```python
from build123d import *

# Parameters (mm, degrees)
SKIZZE1_W                       = 188
SKIZZE1_H                       = 158
AUFSATZ_LINEAR_AUSTRAGEN1_DEPTH = 39
SKIZZE2_W                       = 180
SKIZZE2_H                       = 150
SCHNITT_LINEAR_AUSTRAGEN1_DEPTH = 35
SKIZZE3_W                       = 8
SKIZZE3_H                       = 40
AUFSATZ_LINEAR_AUSTRAGEN2_DEPTH = 30
VERRUNDUNG1_R                   = 20
SKIZZE4_R                       = 5
SCHNITT_LINEAR_AUSTRAGEN2_DEPTH = 208
VERRUNDUNG2_R                   = 10


with BuildPart() as part:
    # Skizze1 → Aufsatz-Linear austragen1 (new body)
    with BuildSketch(Plane.XY):
        Rectangle(SKIZZE1_W, SKIZZE1_H)
    extrude(amount=AUFSATZ_LINEAR_AUSTRAGEN1_DEPTH)

    # Skizze2 → Schnitt-Linear austragen1 (cut)
    with BuildSketch(Plane.XY):
        Rectangle(SKIZZE2_W, SKIZZE2_H)
    extrude(amount=SCHNITT_LINEAR_AUSTRAGEN1_DEPTH, mode=Mode.SUBTRACT)

    # Skizze3 → Aufsatz-Linear austragen2 (add)
    with BuildSketch(Plane.XY.offset(39)):
        with Locations((-90, 0)):
            Rectangle(SKIZZE3_W, SKIZZE3_H)
        Polygon((-34, 20), (-26, 20), (-26, -20), (26, -20), (26, 20), (34, 20), (34, -20), (34, -28), (-34, -28), (-34, -20), align=None)
        with Locations((90, 0)):
            Rectangle(SKIZZE3_W, SKIZZE3_H)
    extrude(amount=AUFSATZ_LINEAR_AUSTRAGEN2_DEPTH)

    # Verrundung1
    verrundung1_edges = [part.edges().sort_by_distance(p)[0] for p in [
        (-90, -20, 69),
        (-90, 20, 69),
        (30, 20, 69),
        (-30, 20, 69),
        (90, -20, 69),
        (90, 20, 69),
    ]]
    fillet(verrundung1_edges, radius=VERRUNDUNG1_R - 0.0001)  # a hair under: the kernel refuses the full size

    # Skizze4 → Schnitt-Linear austragen2 (cut)
    with BuildSketch(Plane.ZY.offset(94)):
        with Locations((54, 0)):
            Circle(SKIZZE4_R)
    extrude(amount=-SCHNITT_LINEAR_AUSTRAGEN2_DEPTH, mode=Mode.SUBTRACT)

    # Verrundung2
    verrundung2_edges = [part.edges().sort_by_distance(p)[0] for p in [
        (-90, 20, 39),
        (-90, -20, 39),
        (90, 20, 39),
        (90, -20, 39),
    ]]
    fillet(verrundung2_edges, radius=VERRUNDUNG2_R)


solid = part.part
```
Source: CAD feature listing. Evaluate the final solid. Frame: model axes, mm. A direction names the side the tool comes from. Give positions to 0.01 mm unless a question says otherwise; leave off trailing zeros. Write each loop counter-clockwise with the first axis right and the second up, starting at its lowest first coordinate (ties: lowest second). Pieces come first, ordered by that corner, then holes.
1. Section query C-C (z = 28.5). Return the cut outline in (x, y).
2. Pull-direction query (Y, two-part tool) for faces 5 (the face through (-94, -1, 26)), 6 (the face through (90.06, -23.01, 41.85)), 7 (the face through (-1, 1, 35)); classes: +Y half, -Y half, draft (parallel to the pull), parting line (faces both ways), or undercut.
3. Section query A-A (z = 54). Count the separate pieces of the cut face and the enclosed holes in it, then the cut area to 3 significant figures.
4. First-contact query: pin 1 (4 mm diameter, centred on x = -31.5, z = 42, fed in from +Y); pin 2 (15 mm diameter, centred on x = -1.5, z = 54.5, fed in from +Y); pin 3 (3 mm diameter, centred on x = 27.5, y = -60, fed in from +Z). Flat tips, straight axial feed; report the tip coordinate or a pass-through.
5. Section query B-B (x = 41). Return the cut outline in (y, z).
6. Section query D-D (y = -64.5). Return the cut outline in (x, z), then the cut area to 3 significant figures.
7. Material intervals for line 1 along X through (y, z) = (9.5, 40); line 2 along Y through (x, z) = (14, 26.5); line 3 along X through (y, z) = (-70, 11.5), sorted ascending.
8. Access query for faces 1 (the face through (-89.94, -22.85, 42.01)), 2 (the face through (-34, -4, 50)), 3 (the face through (-1, 75, 17)), 4 (the face through (-30, 20, 44)). Directions: +Z, -Z, +X, -X, +Y, -Y. A direction counts if a zero-diameter tool reaches every point of the face in a straight line with its end or side. Return the directions, or none.
Output values:
1. outline: (-94, -79) - (94, -79) - (94, 79) - (-94, 79) - close; hole (-90, -75) - (90, -75) - (90, 75) - (-90, 75) - close
2. face 5: draft
2. face 6: -Y half
2. face 7: undercut
3. separate pieces: 7
3. enclosed holes: 0
3. area: 1,470 mm2
4. pin 1: stops at y = 20
4. pin 2: stops at y = -20
4. pin 3: stops at z = 39
5. outline: (-79, 0) - (-75, 0) - (-75, 35) - (75, 35) - (75, 0) - (79, 0) - (79, 39) - (-79, 39) - close
6. outline: (-94, 0) - (-90, 0) - (-90, 35) - (90, 35) - (90, 0) - (94, 0) - (94, 39) - (-94, 39) - close
6. area: 1,030 mm2
7. line 1: x = -94 to -86, -34 to -26, 26 to 34, 86 to 94
7. line 2: y = -79 to -75, 75 to 79
7. line 3: x = -94 to -90, 90 to 94
8. face 1: +Z, -X, -Y
8. face 2: +Z, +Y, -Y
8. face 3: -Z
8. face 4: +Z, +Y
